```python
from build123d import *

# Parameters (mm, degrees)
BOSS_EXTRUDE1_DEPTH         = 28.575
BOSS_EXTRUDE2_DEPTH         = 12.7
BOSS_EXTRUDE2_DEPTH_BACK    = 41.275
SKETCH2_R                   = 6.858
F_1_4_0_25_DIAMETER_HOLE1_D = 6.35
BOSS_EXTRUDE3_DEPTH         = 5.499261
BOSS_EXTRUDE3_DEPTH_BACK    = 5.499261
CUT_EXTRUDE2_DEPTH          = 0.635
SKETCH8_R                   = 3.175
BOSS_EXTRUDE4_DEPTH         = 0.254
DOME1_FACE_RADIUS           = 3.175
DOME1_HEIGHT                = 1.778
CUT_EXTRUDE3_REACH          = 59.165
CUT_EXTRUDE3_END_RADIUS     = 3.723821429
CUT_EXTRUDE3_START          = 0.508
BOSS_EXTRUDE5_REACH         = 58.328
SKETCH10_R                  = 1.5875


with BuildPart() as part:
    # Sketch1 → Boss-Extrude1 (new body)
    with BuildSketch(Plane(origin=(0, 0, 0), x_dir=(0, 0, -1), z_dir=(1, 0, 0))):
        Polygon((10.998522628, 0), (5.499261314, 9.525), (-5.499261314, 9.525), (-10.998522628, 0), (-5.499261314, -9.525), (5.499261314, -9.525), align=None)
    extrude(amount=BOSS_EXTRUDE1_DEPTH)

    # Sketch2 → Boss-Extrude2 (add, two sides: drawn at the far end of the back side and taken through both)
    with BuildSketch(Plane(origin=(28.575, 0, 0), x_dir=(0, 0, -1), z_dir=(1, 0, 0)).offset(-BOSS_EXTRUDE2_DEPTH_BACK)):
        Circle(SKETCH2_R)
    extrude(amount=BOSS_EXTRUDE2_DEPTH + BOSS_EXTRUDE2_DEPTH_BACK)

    # 1/4 (0.25) Diameter Hole1 (through all)
    with Locations(Plane.ZY.offset(12.7)):
        with Locations((0, 0)):
            Hole(F_1_4_0_25_DIAMETER_HOLE1_D / 2)


with BuildPart() as body_2:
    # Sketch6 → Boss-Extrude3 (new, two sides: drawn at the far end of the back side and taken through both)
    with BuildSketch(Plane.XY.offset(-BOSS_EXTRUDE3_DEPTH_BACK)):
        with BuildLine():
            Line((2.54, 9.8425), (15.24, 9.8425))
            ThreePointArc((15.24, 9.8425), (16.181122428, 9.98518841), (17.037654453, 10.400428456))
            Line((17.037654453, 10.400428456), (24.657654453, 15.634571544))
            ThreePointArc((24.657654453, 15.634571544), (25.514186479, 16.04981159), (26.455308906, 16.1925))
            Line((26.455308906, 16.1925), (51.855308906, 16.1925))
            Line((51.855308906, 16.1925), (51.855308906, 16.8275))
            Line((51.855308906, 16.8275), (26.455308906, 16.8275))
            ThreePointArc((26.455308906, 16.8275), (25.325961993, 16.656273907), (24.298123563, 16.157985853))
            Line((24.298123563, 16.157985853), (16.678123563, 10.923842765))
            ThreePointArc((16.678123563, 10.923842765), (15.992897942, 10.591650728), (15.24, 10.4775))
            Line((15.24, 10.4775), (2.54, 10.4775))
            Line((2.54, 10.4775), (2.54, 9.8425))
        make_face()
    extrude(amount=BOSS_EXTRUDE3_DEPTH + BOSS_EXTRUDE3_DEPTH_BACK)

    # Sketch7 → Cut-Extrude2 (cut)
    with BuildSketch(Plane(origin=(0, 10.4775, 0), x_dir=(1, 0, 0), z_dir=(0, 1, 0))):
        with BuildLine():
            Line((2.54, 5.499261314), (2.54, 0))
            ThreePointArc((2.54, 0), (3.390738686, 3.175), (5.715, 5.499261314))
            Line((5.715, 5.499261314), (2.54, 5.499261314))
        make_face()
        with BuildLine():
            Line((2.54, 0), (2.54, -5.499261314))
            Line((2.54, -5.499261314), (5.715, -5.499261314))
            ThreePointArc((5.715, -5.499261314), (3.390738686, -3.175), (2.54, 0))
        make_face()
    extrude(amount=-CUT_EXTRUDE2_DEPTH, mode=Mode.SUBTRACT)

    # Sketch8 → Boss-Extrude4 (add)
    with BuildSketch(Plane(origin=(0, 10.4775, 0), x_dir=(1, 0, 0), z_dir=(0, 1, 0))):
        with Locations(Location((8.89, 0, 0), (0, 0, 270))):
            Circle(SKETCH8_R)
    extrude(amount=BOSS_EXTRUDE4_DEPTH)

    # Dome1: a dome of height H over a round flat face of radius A is a cap of a sphere of radius (A * A + H * H) / (2 * H)
    dome1_r = (DOME1_FACE_RADIUS * DOME1_FACE_RADIUS + DOME1_HEIGHT * DOME1_HEIGHT) / (2 * DOME1_HEIGHT)
    dome1_base = Plane((8.89, 10.7315, 0), z_dir=(0, 1, 0))
    with Locations(dome1_base.offset(DOME1_HEIGHT - dome1_r)):
        dome1_ball = Sphere(dome1_r, mode=Mode.PRIVATE)
    add(split(dome1_ball, bisect_by=dome1_base, keep=Keep.TOP, mode=Mode.PRIVATE))

    # Cut-Extrude3: up to this sphere (the profile starts inside it)
    cut_extrude3_end = Location((8.89, 8.785678571, 0)) * Sphere(CUT_EXTRUDE3_END_RADIUS, mode=Mode.PRIVATE)
    # Sketch9 → Cut-Extrude3 (cut, up to the surface)
    with BuildSketch(Plane(origin=(0, 10.4775, 0), x_dir=(1, 0, 0), z_dir=(0, 1, 0)).offset(CUT_EXTRUDE3_START), mode=Mode.PRIVATE) as cut_extrude3_sk1:
        Polygon((8.5725, 1.5875), (9.2075, 1.5875), (9.2075, 0.3175), (10.4775, 0.3175), (10.4775, -0.3175), (9.2075, -0.3175), (9.2075, -1.5875), (8.5725, -1.5875), (8.5725, -0.3175), (7.3025, -0.3175), (7.3025, 0.3175), (8.5725, 0.3175), align=None)
    cut_extrude3_tool1 = extrude(cut_extrude3_sk1.sketch, amount=CUT_EXTRUDE3_REACH, mode=Mode.PRIVATE) & cut_extrude3_end
    add(cut_extrude3_tool1.solids().sort_by_distance((8.89, 10.9855, 0))[0], mode=Mode.SUBTRACT)

    # Sketch10 → Boss-Extrude5 (add, up to next)
    with BuildSketch(Plane(origin=(0, 9.525, 0), x_dir=(1, 0, 0), z_dir=(0, 1, 0)), mode=Mode.PRIVATE) as boss_extrude5_sk1:
        with Locations(Location((8.89, 0, 0), (0, 0, 90))):
            Circle(SKETCH10_R)
    boss_extrude5_tool1 = extrude(boss_extrude5_sk1.sketch, amount=BOSS_EXTRUDE5_REACH, mode=Mode.PRIVATE) - body_2.part

    add(part.part)  # Boss-Extrude5 merges part
    add(boss_extrude5_tool1.solids().sort_by_distance((8.89, 9.525, 0))[0])


solid = body_2.part
```
Design review of the part built by this model. Coordinates are the model's own, in mm. A direction names the side the tool comes from. Give positions to 0.01 mm unless a question says otherwise; leave off trailing zeros. Write each loop counter-clockwise with the first axis right and the second up, starting at its lowest first coordinate (ties: lowest second). Pieces come first, ordered by that corner, then holes. Notation, with made-up numbers: (88.25, -27) -> (116.25, -27) arc R25 cw to (116.25, -15) -> close; hole circle Ø11 at (0, 22). An arc over 180 degrees is marked (long way). Answer in a Markdown table with one row per item.
(1) Clearance check with flat-ended pins moving along their axes: pin 1 (0.7 mm diameter, centred on y = 11.5, z = 0, fed in from +X); pin 2 (1 mm diameter, centred on x = -2, z = -2.5, fed in from +Y); pin 3 (1.5 mm diameter, centred on y = -3, z = 4.5, fed in from +X) (3 decimals); pin 4 (2 mm diameter, centred on x = 39.5, y = 14.5, fed in from -Z). State where each tip first meets the part, or that it passes through.
Results:
| item | result |
|---|---|
| pin 1 | x = 19.15 |
| pin 2 | y = 6.56 |
| pin 3 | x = 41.275 |
| pin 4 | through |
(2) Consider section A-A (x = 14.5). Count the separate pieces of the cut face and the enclosed holes in it, then the cut area to 3 significant figures.
Results:
| item | result |
|---|---|
| separate pieces | 2 |
| enclosed holes | 1 |
| area | 290 mm2 |
(3) For faces 1 (the flat face through (41.275, 2, -3)), 2 (the flat face through (9.208, 12, -1)), 3 (the flat face through (30.4, 16.5, -5.499)), 4 (the flat face through (0, 0.1, -7.2)), list the 3-axis set-ups (+Z, -Z, +X, -X, +Y, -Y) from which the entire face can be reached by the end or side of a thin tool; tool diameter is ignored.
Results:
| item | result |
|---|---|
| face 1 | +Z, -Z, +X, -Y |
| face 2 | +Y |
| face 3 | -Z, +X, -X, +Y |
| face 4 | -X |
(4) To check wall thickness, follow probe 1 along Y at (x, z) = (30.5, 0) (1 decimal); probe 2 along Y at (x, z) = (5, 0) (1 decimal); probe 3 along Y at (x, z) = (8.5, 0) (1 decimal). State the ranges of each line that lie inside material, in increasing order.
Results:
| item | result |
|---|---|
| probe 1 | -6.9 to -3.2, 3.2 to 6.9, 16.2 to 16.8 |
| probe 2 | -9.5 to -3.2, 3.2 to 9.5, 9.8 to 10.5 |
| probe 3 | -9.5 to -3.2, 3.2 to 11 |
(5) Consider section D-D (x = -9). State the section outline as (y, z) points (3 decimals), then the cut area to 3 significant figures.
Results:
| item | result |
|---|---|
| outline | circle Ø13.716 at (0, 0); hole circle Ø6.35 at (0, 0) |
| area | 116 mm2 |
(6) Mouldability with a two-part tool opening along X and no side actions: class faces 5 (the cylindrical face through (7.316, 9.682, 0.207)), 6 (the flat face through (10, 12, 0.318)), 7 (the flat face through (14.09, 4.83, 8.21)), 8 (the flat face through (9, 10.985, 0)) as +X half, -X half, draft (parallel to the pull), parting line (faces both ways), or undercut.
Results:
| item | result |
|---|---|
| face 5 | parting line |
| face 6 | undercut |
| face 7 | draft |
| face 8 | undercut |
